from build123d import *

# Parameters (mm, degrees)
SKETCH_1_R          = 1.5
EXTRUDE_2_DEPTH     = 30
SKETCH_2_R          = 1.5
CUT_EXTRUDE_1_DEPTH = 216.996068062


with BuildPart() as part:
    # 草图1 → 凸台-拉伸2 (new body)
    with BuildSketch(Plane.XY):
        with BuildLine():
            Line((23.003941811, 212.114539339), (0.015767245, 30.124824021))
            ThreePointArc((0.015767245, 30.124824021), (0.003945703, 29.999751784), (0, 29.874184094))
            Line((0, 29.874184094), (0, 2))
            ThreePointArc((0, 2), (0.585786438, 0.585786438), (2, 0))
            Line((2, 0), (22, 0))
            ThreePointArc((22, 0), (23.414213562, 0.585786438), (24, 2))
            Line((24, 2), (24, 212.051879357))
            ThreePointArc((24, 212.051879357), (23.531391922, 212.550892931), (23.003941811, 212.114539339))
        make_face()
        with Locations((20, 3)):
            Circle(SKETCH_1_R, mode=Mode.SUBTRACT)
        with Locations((4, 3)):
            Circle(SKETCH_1_R, mode=Mode.SUBTRACT)
        with Locations((20, 19)):
            Circle(SKETCH_1_R, mode=Mode.SUBTRACT)
    extrude(amount=EXTRUDE_2_DEPTH)

    # 草图2 → 切除-拉伸1 (cut, through all)
    with BuildSketch(Plane(origin=(0, 0, 0), x_dir=(-1, 0, 0), z_dir=(0, 0, -1))):
        with Locations((-20, 79)):
            Circle(SKETCH_2_R)
    extrude(amount=-CUT_EXTRUDE_1_DEPTH, mode=Mode.SUBTRACT)


solid = part.part
Check sheet for the modelled part. Datum: model origin and axes. Units: mm. Coordinates: 2 decimals unless noted, no trailing zeros. Write each loop counter-clockwise with the first axis right and the second up, starting at its lowest first coordinate (ties: lowest second). Pieces come first, ordered by that corner, then holes. Notation, with made-up numbers: M 38,-21 L 69,-21 A10 cw 69,-3 Z; hole C 31.5,30.25 d11. An arc over 180 degrees is marked long. Answer as CSV lines item,"result".
Q1. Cross-section at C-C (x = 8). Record the boundary of the cut face in (y, z), then the cut area to 3 significant figures.
Check result:
outline,"M 0,0 L 93.33,0 L 93.33,30 L 0,30 Z"
area,"2,800 mm^2"
Q2. Material ranges on probe 1 along X at (y, z) = (50, 28.5); probe 2 along X at (y, z) = (79, 20.25); probe 3 along X at (y, z) = (80, 5.75), recorded low to high. Write a range as from..to.
Check result:
probe 1,"2.53..24"
probe 2,"6.19..18.5, 21.5..24"
probe 3,"6.32..18.88, 21.12..24"
Q3. Cross-section at A-A (z = 23). Record the boundary of the cut face in (x, y).
Check result:
outline,"M 0,2 A2 ccw 2,0 L 22,0 A2 ccw 24,2 L 24,212.05 A0.5 ccw 23,212.11 L 0.02,30.12 A2 ccw 0,29.87 Z; hole C 4,3 d3; hole C 20,3 d3; hole C 20,19 d3; hole C 20,79 d3"
Q4. Cross-section at B-B (y = 43). Record the boundary of the cut face in (x, z).
Check result:
outline,"M 1.64,0 L 24,0 L 24,30 L 1.64,30 Z"
